from build123d import *

# Parameters (mm, degrees)
SKETCH1_R           = 0.762
BOSS_EXTRUDE1_DEPTH = 1.524
SKETCH2_W           = 12.7
SKETCH2_H           = 0.641845345
BOSS_EXTRUDE2_DEPTH = 5.08
FILLET1_R           = 0.508
CIRPATTERN1_START   = -13.97
CIRPATTERN1_DEPTH   = 12.7
CIRPATTERN1_2_DEPTH = 12.7


# Read off the part's stored shape, not the designer's step: CirPattern1
with BuildPart() as part:
    # Sketch1 → Boss-Extrude1 (new body)
    with BuildSketch(Plane(origin=(0, 0, 0), x_dir=(1, 0, 0), z_dir=(0, 1, 0))):
        with BuildLine():
            Line((1.27, 0), (14.478, 0))
            ThreePointArc((14.478, 0), (12.127384736, 7.908161825), (5.838820078, 13.248421193))
            Line((5.838820078, 13.248421193), (0.5121772, 1.16214221))
            ThreePointArc((0.5121772, 1.16214221), (-0.068857603, 1.268131945), (-0.635, 1.099852263))
            Line((-0.635, 1.099852263), (-7.239, 12.538315796))
            ThreePointArc((-7.239, 12.538315796), (-12.912361406, 6.548542351), (-14.392879352, -1.56764408))
            Line((-14.392879352, -1.56764408), (-1.262533276, -0.137512639))
            ThreePointArc((-1.262533276, -0.137512639), (-1.063805679, -0.693698406), (-0.635, -1.099852263))
            Line((-0.635, -1.099852263), (-7.239, -12.538315796))
            ThreePointArc((-7.239, -12.538315796), (0.78497667, -14.456704176), (8.554059274, -11.680777112))
            Line((8.554059274, -11.680777112), (0.750356077, -1.024629571))
            ThreePointArc((0.750356077, -1.024629571), (1.132663281, -0.57443354), (1.27, 0))
        make_face()
        with Locations(Location((0, 0, 0), (0, 0, 90))):
            Circle(SKETCH1_R, mode=Mode.SUBTRACT)
        with BuildLine():
            ThreePointArc((13.091283697, 2.537817206), (12.588737673, 1.793574306), (11.844494773, 2.296120329))
            ThreePointArc((11.844494773, 2.296120329), (10.203630871, 6.438178474), (7.171403907, 9.702329153))
            ThreePointArc((7.171403907, 9.702329153), (7.038197315, 10.590420367), (7.926288529, 10.723626959))
            ThreePointArc((7.926288529, 10.723626959), (11.277697278, 7.115881471), (13.091283697, 2.537817206))
        make_face(mode=Mode.SUBTRACT)
        with BuildLine():
            ThreePointArc((-4.347827678, -12.606292852), (-4.741087925, -11.79895378), (-3.933748852, -11.405693533))
            ThreePointArc((-3.933748852, -11.405693533), (0.473810677, -12.055692782), (4.816761569, -11.061782541))
            ThreePointArc((4.816761569, -11.061782541), (5.652474417, -11.390467855), (5.323789103, -12.226180703))
            ThreePointArc((5.323789103, -12.226180703), (0.523685485, -13.324713074), (-4.347827678, -12.606292852))
        make_face(mode=Mode.SUBTRACT)
        with BuildLine():
            ThreePointArc((-8.743456019, 10.068475647), (-7.847649749, 10.005379474), (-7.910745922, 9.109573204))
            ThreePointArc((-7.910745922, 9.109573204), (-10.677441547, 5.617514308), (-11.988165476, 1.359453388))
            ThreePointArc((-11.988165476, 1.359453388), (-12.690671732, 0.800047488), (-13.250077632, 1.502553744))
            ThreePointArc((-13.250077632, 1.502553744), (-11.801382763, 6.208831604), (-8.743456019, 10.068475647))
        make_face(mode=Mode.SUBTRACT)
    extrude(amount=BOSS_EXTRUDE1_DEPTH)

    # Sketch2 → Boss-Extrude2 (add)
    with BuildSketch(Plane.XZ):
        with Locations((7.62, -0.320922673)):
            Rectangle(SKETCH2_W, SKETCH2_H)
    extrude(amount=BOSS_EXTRUDE2_DEPTH)

    # Fillet1
    fillet1_edges = [part.edges().sort_by_distance(p)[0] for p in [
        (7.62, 0, -0.641845345),
        (7.874, 1.524, 0),
    ]]
    fillet(fillet1_edges, radius=FILLET1_R)

    # CirPattern1 outline → CirPattern1 (add)
    with BuildSketch(Plane(origin=(0, 0, 0), x_dir=(0.8660254037844362, 0, -0.5000000000000042), z_dir=(0.5000000000000042, 0, 0.8660254037844363)).offset(CIRPATTERN1_START)):
        with BuildLine():
            Line((-0.641845345, -0.508), (-0.641845345, -5.08))
            Line((-0.641845345, -5.08), (0, -5.08))
            Line((0, -5.08), (0, 0))
            Line((0, 0), (-1.149845345, 0))
            ThreePointArc((-1.149845345, 0), (-0.7906351, -0.148789755), (-0.641845345, -0.508))
        make_face()
    extrude(amount=CIRPATTERN1_DEPTH)

    # CirPattern1 2 outline → CirPattern1 2 (add)
    with BuildSketch(Plane(origin=(0, 0, 0), x_dir=(0.8660254037844431, 0, 0.4999999999999921), z_dir=(0.4999999999999921, 0, -0.8660254037844433)).offset(CIRPATTERN1_START)):
        with BuildLine():
            Line((0.641845345, 0.508), (0.641845345, 5.08))
            Line((0.641845345, 5.08), (0, 5.08))
            Line((0, 5.08), (0, 0))
            Line((0, 0), (1.149845345, 0))
            ThreePointArc((1.149845345, 0), (0.7906351, 0.148789755), (0.641845345, 0.508))
        make_face()
    extrude(amount=CIRPATTERN1_2_DEPTH)


solid = part.part
For this review, take the finished solid that the model builds, in its own axes (mm). A direction names the side the tool comes from. Round coordinates to 2 decimals unless told otherwise and drop trailing zeros. Order: outer loops, then holes, each group sorted by start corner. A loop starts at its lowest first (then second) coordinate and runs counter-clockwise, first axis right, second up. Notation, with made-up numbers: (71, -21.5) -> (99, -21.5) arc R16 cw to (99, 4.5) -> close; hole circle Ø1 at (-37.75, 45). An arc over 180 degrees is marked (long way). Write item = value, one per line. Start each with the question number.
1) Take a section at A-A on y = -2. State the section outline as (x, z) points (3 decimals), plus the area to 3 significant figures.
2) Take a section at B-B on x = 7.5. State the section outline as (y, z) points.
3) Tool access review of faces 1 (the face through (-11.83, 0.75, -6.15)), 2 (the face through (8, -3, -0.642)), 3 (the face through (4.71, 0.75, 6.43)): name each direction out of +Z, -Z, +X, -X, +Y, -Y from which nothing blocks a thin tool from reaching the whole face with its end or side.
4) Take a section at C-C on x = 3.75. State the section outline as (y, z) points.
5) The part is to be moulded in two halves that separate along X. For faces 4 (the face through (-12.7, 0.8, -0.8)), 5 (the face through (-4.41, -2.762, -6.355)), 6 (the face through (8, -2, 0)), say which applies: +X half, -X half, draft (parallel to the pull), parting line (faces both ways), or undercut.
6) Take a section at D-D on z = -4.5. Count the separate pieces of the cut face and the enclosed holes in it, plus the area to 3 significant figures.
7) Insertion check: pin 1 (2 mm diameter, centred on x = 11.5, y = -1, fed in from +Z); pin 2 (3 mm diameter, centred on x = 5.5, z = -7.5, fed in from -Y); pin 3 (3.5 mm diameter, centred on x = 8, y = -2, fed in from -Z); pin 4 (0.9 mm diameter, centred on x = 0, z = 0, fed in from -Y). Each pin has a flat end and moves straight along its axis. Give the tip position at first contact, or say it passes through.
8) To check wall thickness, follow line 1 (X direction, y = 1.2, z = 0); line 2 (Y direction, x = 3, z = 6.25); line 3 (Z direction, x = 8, y = 0.5). State the ranges of each line that lie inside material, in increasing order. Write a range as from..to.
Verdict:
q1.outline = (-7.541, -11.777) -> (-6.985, -12.098) -> (-0.635, -1.1) -> (-1.191, -0.779) -> close; (-6.985, 12.098) -> (-0.635, 1.1) -> (-0.079, 1.421) -> (-6.429, 12.419) -> close; (1.27, -0.642) -> (13.97, -0.642) -> (13.97, 0) -> (1.27, 0) -> close
q1.area = 24.5 mm2
q2.outline = (-5.08, -0.64) -> (-0.51, -0.64) arc R0.51 cw to (0, -1.15) -> (0, -9.45) -> (1.52, -9.45) -> (1.52, -0.51) arc R0.51 ccw to (1.02, 0) -> (-5.08, 0) -> close; (0, -12.38) -> (1.52, -12.38) -> (1.52, -10.85) -> (0, -10.85) -> close; (0, 10.24) -> (1.52, 10.24) -> (1.52, 12.38) -> (0, 12.38) -> close
q3.face_1 = +Y, -Y
q3.face_2 = -Z, +X, -X, -Y
q3.face_3 = +X, +Y, -Y
q4.outline = (-5.08, -0.64) -> (-0.51, -0.64) arc R0.51 cw to (0, -1.15) -> (0, -8.51) -> (1.52, -8.51) -> (1.52, -0.51) arc R0.51 ccw to (1.02, 0) -> (-5.08, 0) -> close; (0, 5.12) -> (1.52, 5.12) -> (1.52, 11.47) -> (0, 11.47) -> close; (0, 12.8) -> (1.52, 12.8) -> (1.52, 13.98) -> (0, 13.98) -> close
q5.face_4 = undercut
q5.face_5 = -X half
q5.face_6 = draft
q6.separate_pieces = 4
q6.enclosed_holes = 0
q6.area = 34.6 mm2
q7.pin_1 = 0
q7.pin_2 = 0
q7.pin_3 = -0.71
q7.pin_4 = through
q8.line_1 = -14.48..-0.76, 0.76..1.27
q8.line_2 = 0..1.52
q8.line_3 = -12.07..-10.67, -9.03..0, 10.92..12.07
